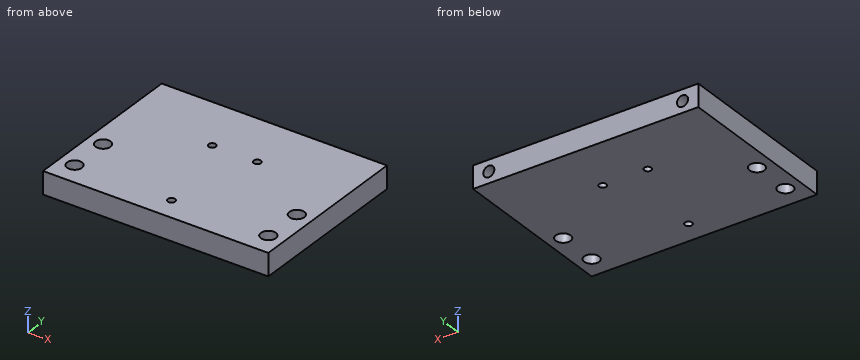
Autodesk Inventor part; units mm, degrees
ref_plane "YZ Plane" through (0, 0, 0) normal (1, 0, 0) x (0, 1, 0)
ref_plane "XZ Plane" through (0, 0, 0) normal (0, 1, 0) x (-1, 0, 0)
ref_plane "XY Plane" through (0, 0, 0) normal (0, 0, 1) x (1, 0, 0)
sketch "Sketch1" plane through (0, 0, 0) normal (0, 0, 1) x (1, 0, 0)
  line L0 (50, -30) -> (-50, -30)
  line L1 (-50, -30) -> (-50, 30)
  line L2 (-50, 30) -> (50, 30)
  line L3 (50, 30) -> (50, -30)
  line L4 (50, -30) -> (-50, 30) construction
  line L5 (-50, -30) -> (50, 30) construction
  line L6 (-70, 0) -> (70, 0)
  line L7 (-50, 30) -> (50, 30)
  line L8 (50, 30) -> (50, 45)
  line L9 (50, 45) -> (-50, 45)
  line L10 (-50, 45) -> (-50, 30)
  point P0 (0, 0)
  dimension "d2" = 100
  dimension "d3" = 60
  dimension "d45" = 15
extrude "Extrusion1" add sketch "Sketch1" along normal blind 10 contours L0 L1 L6 L3 | L6 L1 L2 L3
sketch "Sketch2" plane through (0, 0, 10) normal (0, 0, 1) x (1, 0, 0)
  line L0 (-43, -20) -> (43, -20) construction
  line L1 (43, -20) -> (43, -2) construction
  line L2 (43, -2) -> (-43, -2) construction
  line L3 (-43, -2) -> (-43, -20) construction
  line L4 (-50, -30) -> (50, -30) construction
  line L5 (0, -42) -> (0, 42) construction
  point P0 (0, 0)
  dimension "d6" = 86
  dimension "d7" = 18
  dimension "d8" = 10
hole "Hole1" at (-43, -2, 10) at (43, -2, 10) at (43, -20, 10) at (-43, -20, 10) direction (0, 0, -1) diameter 6.647 end through all
sketch "Sketch3" plane through (0, 0, 10) normal (0, 0, 1) x (1, 0, 0)
  line L0 (50, 30) -> (-50, 30)
  line L1 (0, -42) -> (0, 42)
  point P0 (0, 0)
  point P1 (-10, 20)
  point P2 (10, 20)
  point P3 (0, -20)
  dimension "d16" = 10
  dimension "d17" = 10
  dimension "d18" = 40
hole "Hole4" at (-10, 20, 10) at (10, 20, 10) at (0, -20, 10) direction (0, 0, -1) diameter 3.242 end through all
extrude "Extrusion3" add sketch "Sketch1" along normal blind 10 contours L2 L10 L9 L8
sketch "Sketch5" plane through (-50, 45, 0) normal (0, 1, 0) x (1, 0, 0)
  line L0 (0, -10) -> (100, -10) construction
  line L1 (50, -10) -> (50, 0) construction
  line L2 (48.379, 0) -> (48.379, -10) construction
  point P0 (93, -5)
  point P1 (7, -5)
  dimension "d48" = 5
  dimension "d49" = 86
hole "Hole5" at (43, 45, 5) at (-43, 45, 5) direction (0, -1, 0) diameter 4.917 depth 15 tip angle 118
properties part number "Lift_adaptor" material "Stainless Steel"
Read the model definition and answer for the solid it produces. Units are mm, in the model's axes. Give positions to 0.01 mm unless a question says otherwise; leave off trailing zeros. Order: outer loops, then holes, each group sorted by start corner. A loop starts at its lowest first (then second) coordinate and runs counter-clockwise, first axis right, second up. Notation, with made-up numbers: (-34, 62) -> (23, 62) arc R14 ccw to (23, 66) -> close; hole circle Ø5 at (70, 22.5). An arc over 180 degrees is marked (long way). One line per item, written item: value. Start each with the question number.
(1) The part is cut by section A-A (y = -2). Determine the outline of the cut face in (x, z), and give its area (3 significant figures).
(2) The part is cut by section B-B (x = -10). Determine the outline of the cut face in (y, z).
(3) Flat-ended cylindrical pins translate along their axes: P1, Ø1.9, axis at x = 10, y = 20, coming from the +Z side; P2, Ø3, axis at x = 43, z = 5, coming from the +Y side. Find the tip coordinate at first contact, or state that the pin passes through.
(4) The part is cut by section D-D (y = 36). Determine the outline of the cut face in (x, z).
(5) Straight lines are drawn through the part: L1, parallel to X at y = 34, z = 5; L2, parallel to X at y = 20, z = 6; L3, parallel to Z at x = -43, y = 36.25. For each, find the intervals that lie inside material, in ascending order.
(6) The part is cut by section C-C (z = 8.5). Determine the outline of the cut face in (x, y), and give its area (3 significant figures).
Taken from the geometry:
1. outline: (-50, 0) -> (-46.32, 0) -> (-46.32, 10) -> (-50, 10) -> close; (-39.68, 0) -> (39.68, 0) -> (39.68, 10) -> (-39.68, 10) -> close; (46.32, 0) -> (50, 0) -> (50, 10) -> (46.32, 10) -> close
1. area: 867 mm^2
2. outline: (-30, 0) -> (18.38, 0) -> (18.38, 10) -> (-30, 10) -> close; (21.62, 0) -> (45, 0) -> (45, 10) -> (21.62, 10) -> close
3. P1: through
3. P2: y = 29.42
4. outline: (-50, 0) -> (50, 0) -> (50, 10) -> (-50, 10) -> close; hole circle Ø4.92 at (-43, 5); hole circle Ø4.92 at (43, 5)
5. L1: -50 to -45.46, -40.54 to 40.54, 45.46 to 50
5. L2: -50 to -11.62, -8.38 to 8.38, 11.62 to 50
5. L3: 0 to 2.54, 7.46 to 10
6. outline: (-50, -30) -> (50, -30) -> (50, 45) -> (-50, 45) -> close; hole circle Ø6.65 at (-43, -20); hole circle Ø6.65 at (-43, -2); hole circle Ø3.24 at (-10, 20); hole circle Ø3.24 at (0, -20); hole circle Ø3.24 at (10, 20); hole circle Ø6.65 at (43, -20); hole circle Ø6.65 at (43, -2)
6. area: 7,340 mm^2
